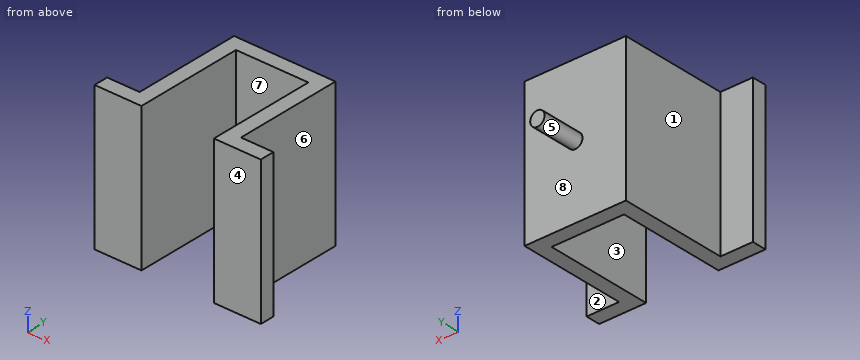
from build123d import *

# Parameters (mm, degrees)
BOSS_EXTRUDE1_DEPTH   = 100
BOSS_EXTRUDE1_2_DEPTH = 100
SKETCH2_W             = 70
SKETCH2_H             = 100
BOSS_EXTRUDE2_DEPTH   = 10
SKETCH3_R             = 5
BOSS_EXTRUDE3_DEPTH   = 30


with BuildPart() as part:
    # Sketch1 → Boss-Extrude1 (new body)
    with BuildSketch(Plane.XY):
        Polygon((-57.404010399, -45.485546177), (-25, -45.485546177), (-25, 29.514453823), (-35, 29.514453823), (-35, -35.485546177), (-57.404010399, -35.485546177), align=None)
    extrude(amount=BOSS_EXTRUDE1_DEPTH)



with BuildPart() as body_2:
    # Sketch1 → Boss-Extrude1 2 (new body)
    with BuildSketch(Plane.XY):
        Polygon((25, 29.514453823), (35, 29.514453823), (35, -35.485546177), (57.404010399, -35.485546177), (57.404010399, -45.485546177), (25, -45.485546177), align=None)
    extrude(amount=BOSS_EXTRUDE1_2_DEPTH)


with BuildPart() as part_1:
    add(part.part)

    add(body_2.part)  # Boss-Extrude2 merges body 2
    # Sketch2 → Boss-Extrude2 (add)
    with BuildSketch(Plane(origin=(0, 29.514453823, 0), x_dir=(1, 0, 0), z_dir=(0, 1, 0))):
        with Locations((0, -50)):
            Rectangle(SKETCH2_W, SKETCH2_H)
    extrude(amount=BOSS_EXTRUDE2_DEPTH)

    # Sketch3 → Boss-Extrude3 (add)
    with BuildSketch(Plane(origin=(0, 39.514453823, 0), x_dir=(1, 0, 0), z_dir=(0, 1, 0))):
        with Locations(Location((0, -50, 0), (0, 0, 180))):
            Circle(SKETCH3_R)
    extrude(amount=BOSS_EXTRUDE3_DEPTH)


solid = part_1.part
CAD build for the part. Positions are in the model's coordinates, mm. Face numbers are marked on the shaded views. A direction names the side the tool comes from. Give positions to 0.01 mm unless a question says otherwise; leave off trailing zeros. Order: outer loops, then holes, each group sorted by start corner. A loop starts at its lowest first (then second) coordinate and runs counter-clockwise, first axis right, second up. Notation, with made-up numbers: (18, -1.75) - (58, -1.75) arc R21 ccw to (58, 33.25) - close; hole circle Ø1 at (51, 13.5). An arc over 180 degrees is marked (long way). Write each question's results on one line, items separated by ' | '.
1. Saw through at C-C on z = 50. List the corners of the cut face in (x, y).
Calculated:
outline: (-57.4, -45.49) - (-25, -45.49) - (-25, 29.51) - (25, 29.51) - (25, -45.49) - (57.4, -45.49) - (57.4, -35.49) - (35, -35.49) - (35, 39.51) - (5, 39.51) - (5, 69.51) - (-5, 69.51) - (-5, 39.51) - (-35, 39.51) - (-35, -35.49) - (-57.4, -35.49) - close
2. Saw through at D-D on z = 71.5. List the corners of the cut face in (x, y), and give its area (3 significant figures).
Calculated:
outline: (-57.4, -45.49) - (-25, -45.49) - (-25, 29.51) - (25, 29.51) - (25, -45.49) - (57.4, -45.49) - (57.4, -35.49) - (35, -35.49) - (35, 39.51) - (-35, 39.51) - (-35, -35.49) - (-57.4, -35.49) - close | area: 2,650 mm2
3. Pin check, flat tips, straight feed: pin 1 (8 mm diameter, centred on x = -36.5, z = 20.5, fed in from +Y); pin 2 (18 mm diameter, centred on x = -46.5, z = 69, fed in from +Y); pin 3 (1 mm diameter, centred on y = -15.5, z = 26, fed in from -X). Stop position of each tip, or through.
Calculated:
pin 1: stops at y = 39.51 | pin 2: stops at y = -35.49 | pin 3: stops at x = -35
4. Saw through at A-A on y = -19. List the corners of the cut face in (x, z), and give its area (3 significant figures).
Calculated:
outline: (-35, 0) - (-25, 0) - (-25, 100) - (-35, 100) - close; (25, 0) - (35, 0) - (35, 100) - (25, 100) - close | area: 2,000 mm2
5. Pull direction X, two halves, no side cores. Call the marked faces 6, 7 and 8: released by +X, released by -X, zero draft, split by the parting line, or undercut.
Calculated:
face 6: released by +X | face 7: undercut | face 8: zero draft
6. Saw through at B-B on x = 0. List the corners of the cut face in (y, z), and give its area (3 significant figures).
Calculated:
outline: (29.51, 0) - (39.51, 0) - (39.51, 45) - (69.51, 45) - (69.51, 55) - (39.51, 55) - (39.51, 100) - (29.51, 100) - close | area: 1,300 mm2
7. Probe L1, parallel to X at y = 28.5, z = 96.5; L2, parallel to Y at x = -24.5, z = 62; L3, parallel to Y at x = 32, z = 35. List the from-to ranges inside material, lowest first. Write a range as from..to.
Calculated:
L1: x = -35..-25, 25..35 | L2: y = 29.51..39.51 | L3: y = -45.49..39.51
8. 3-axis set-ups, long thin cutter, end or side, ignore diameter. For the marked faces 1, 2, 3, 4 and 5: which of +Z, -Z, +X, -X, +Y, -Y reach the whole face in a straight line?
Calculated:
face 1: +Z, -Z, -X, +Y | face 2: +Z, -Z, +X, +Y | face 3: +Z, -Z, -Y | face 4: +Z, -Z, +X, -X, -Y | face 5: +Y
